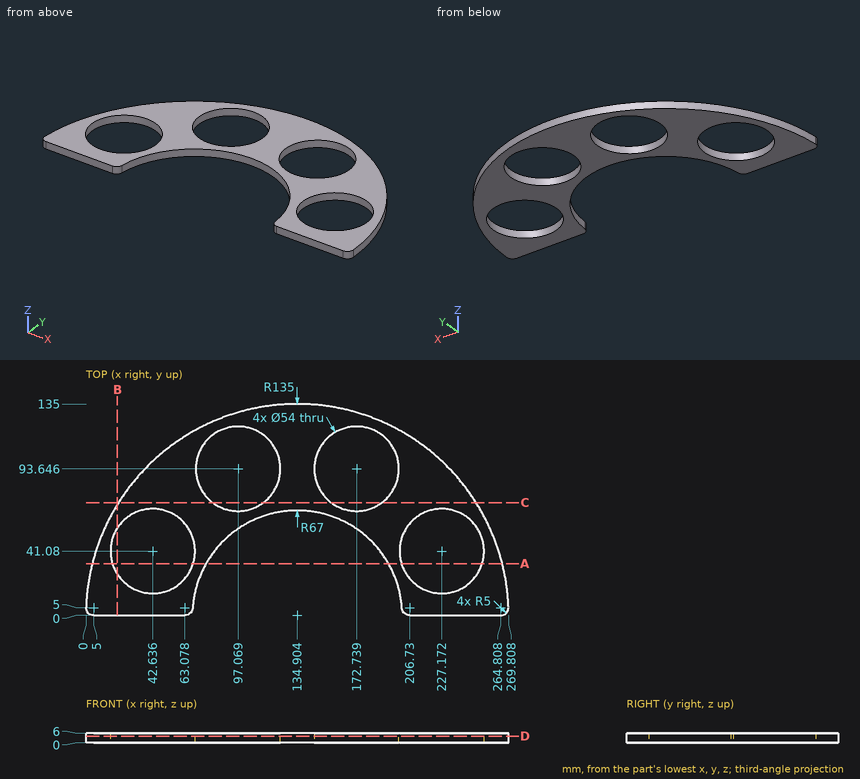
Part print with two shaded views. Sizes in mm from the minimum x, y, z corner. Coordinates: 2 decimals unless noted, no trailing zeros. Order: outer loops, then holes, each group sorted by start corner. A loop starts at its lowest first (then second) coordinate and runs counter-clockwise, first axis right, second up.
(1) Drill centre lines: L1, parallel to X at y = 53, z = 5.1 (1 decimal); L2, parallel to X at y = 51.5, z = 1.7 (1 decimal); L3, parallel to X at y = 114.5, z = 4.5 (1 decimal). Where is each one in solid material? Low to high.
Solution:
L1: x = 10.7 to 18.4, 66.9 to 93.9, 175.9 to 202.9, 251.4 to 259.1
L2: x = 10.1 to 17.7, 67.5 to 92, 177.8 to 202.3, 252.1 to 259.7
L3: x = 63.4 to 79.9, 114.2 to 155.6, 189.9 to 206.4
(2) Saw through at A-A, the plane y = 33. Write the cut outline in (x, z) (1 decimal).
Solution:
outline: (4, 0) - (16.9, 0) - (16.9, 6) - (4, 6) - close; (68.4, 0) - (76.6, 0) - (76.6, 6) - (68.4, 6) - close; (193.2, 0) - (201.4, 0) - (201.4, 6) - (193.2, 6) - close; (252.9, 0) - (265.8, 0) - (265.8, 6) - (252.9, 6) - close
(3) Saw through at C-C, the plane y = 72. Write the cut outline in (x, z), and give its area (3 significant figures).
Solution:
outline: (20.71, 0) - (80.93, 0) - (80.93, 6) - (20.71, 6) - close; (113.21, 0) - (156.6, 0) - (156.6, 6) - (113.21, 6) - close; (188.88, 0) - (249.1, 0) - (249.1, 6) - (188.88, 6) - close
area: 983 mm2
(4) Pin check, flat tips, straight feed: pin 1 Ø2 at (x, z) = (168, 1.5) entering from +Y; pin 2 Ø3 at (x, z) = (233.5, 3) entering from -Y; pin 3 Ø1 at (x, z) = (119, 1.5) entering from -Y; pin 4 Ø2 at (y, z) = (94, 1) entering from -X (1 decimal). Stop position of each tip, or through.
Solution:
pin 1: stops at y = 131.13
pin 2: stops at y = 0
pin 3: stops at y = 64.96
pin 4: stops at x = 37
(5) Saw through at D-D, the plane z = 4.2. Write the cut outline in (x, y) (1 decimal).
Solution:
outline: (0, 5.2) arc R5 ccw to (5, 0) - (63.1, 0) arc R5 ccw to (68.1, 4.7) arc R67 cw to (201.7, 4.7) arc R5 ccw to (206.7, 0) - (264.8, 0) arc R5 ccw to (269.8, 5.2) arc R135 ccw to start; hole circle Ø54 at (42.6, 41.1); hole circle Ø54 at (97.1, 93.6); hole circle Ø54 at (172.7, 93.6); hole circle Ø54 at (227.2, 41.1)
(6) Saw through at B-B, the plane x = 20. Write the cut outline in (y, z).
Solution:
outline: (0, 0) - (26.36, 0) - (26.36, 6) - (0, 6) - close; (55.8, 0) - (70.87, 0) - (70.87, 6) - (55.8, 6) - close
